```python
from build123d import *

# Parameters (mm, degrees)
F0_W     = 152.4
F0_H     = 25.4
F1_DEPTH = 1.778
F1_TAPER = -3


with BuildPart() as f1:
    # F0 (on Top) → F1 (new body, symmetric)
    with BuildSketch(Plane.XY):
        with Locations((0.0009177437, -12.7)):
            Rectangle(F0_W, F0_H)
        with BuildLine():
            Line((-76.1990822563, -25.4), (-76.1990822563, 0))
            Line((-76.1990822563, 0), (-125.9606556381, -10.2188949775))
            ThreePointArc((-125.9606556381, -10.2188949775), (-102.2119643301, -21.5203003803), (-76.1990822563, -25.4))
        make_face()
    extrude(amount=F1_DEPTH, both=True, taper=F1_TAPER)


solid = f1.part
```
Design review of the part built by this model. Coordinates are the model's own, in mm. Give positions to 0.01 mm unless a question says otherwise; leave off trailing zeros. Use a Markdown table: item, result. Add a question column.
(1) Wall thickness on probe 1 along Y at (x, z) = (-37.5, -0.05); probe 2 along Y at (x, z) = (-3.5, -1.6); probe 3 along X at (y, z) = (-11.5, -1.1): over which ranges is each line inside the solid? List them lowest first. Write a range as [from, to].
(2) Clearance check with a flat-ended pin moving along its axis: P1, Ø2, axis at x = -79.5, z = 1, coming from the -Y side. State where the tip first meets the part, or that it passes through.
(3) Mouldability with a two-part tool opening along Z and no side actions: class faces 1 (the face through (-16, -16, -1.778)), 2 (the face through (-16, -16, 1.778)) as +Z half, -Z half, draft (parallel to the pull), parting line (faces both ways), or undercut.
Report:
| question | item | result |
|---|---|---|
| 1 | probe 1 | y = [-25.4, 0] |
| 1 | probe 2 | y = [-25.48, 0.08] |
| 1 | probe 3 | x = [-124.11, 76.26] |
| 2 | P1 | stops at y = -25.45 |
| 3 | face 1 | -Z half |
| 3 | face 2 | +Z half |
